```python
from build123d import *

# Parameters (mm, degrees)
BOSS_EXTRUDE1_DEPTH = 20
BOSS_EXTRUDE2_DEPTH = 10
FILLET1_R           = 3
FILLET2_R           = 1
BOSS_EXTRUDE4_DEPTH = 2
CUT_EXTRUDE1_REACH  = 44.805


with BuildPart() as part:
    # Sketch1 → Boss-Extrude1 (new body)
    with BuildSketch(Plane.XY):
        with BuildLine():
            Line((-11.5, 7), (11.5, 7))
            ThreePointArc((11.5, 7), (18.5, 0), (11.5, -7))
            Line((11.5, -7), (-11.5, -7))
            ThreePointArc((-11.5, -7), (-18.5, 0), (-11.5, 7))
        make_face()
        with BuildLine():
            Line((-11.5, 5), (11.5, 5))
            ThreePointArc((11.5, 5), (16.5, 0), (11.5, -5))
            Line((11.5, -5), (-11.5, -5))
            ThreePointArc((-11.5, -5), (-16.5, 0), (-11.5, 5))
        make_face(mode=Mode.SUBTRACT)
    extrude(amount=BOSS_EXTRUDE1_DEPTH)

    # Sketch2 → Boss-Extrude2 (add)
    with BuildSketch(Plane(origin=(0, 0, 0), x_dir=(-1, 0, 0), z_dir=(0, 0, -1))):
        with BuildLine():
            Line((11.25, -7), (6.75, -7))
            ThreePointArc((6.75, -7), (9.829603655, -12.636154321), (8.962619003, -19))
            Line((8.962619003, -19), (11.25, -19))
            Line((11.25, -19), (11.25, -7))
        make_face()
        with BuildLine():
            Line((-11.25, -19), (-8.962619003, -19))
            ThreePointArc((-8.962619003, -19), (-9.829603655, -12.636154321), (-6.75, -7))
            Line((-6.75, -7), (-11.25, -7))
            Line((-11.25, -7), (-11.25, -19))
        make_face()
    extrude(amount=-BOSS_EXTRUDE2_DEPTH)

    # Fillet1
    # the kernel refuses this fillet: 3 mm, written as the material it adds along each edge
    with BuildSketch(Plane(origin=(-11.25, -7, 0), x_dir=(-0.9923889232111901, 0.12314310816174315, 0), z_dir=(0, 0, 1))) as fillet1_piece_1:
        with BuildLine():
            CenterArc((2.655216223, 2.963972865), FILLET1_R, 187.073535236, 74.037985837)
            Line((-0.321950546, 2.594543541), (-0.619667223, 2.557600608))
            Line((-0.619667223, 2.557600608), (-0.297716677, -0.036942932))
            Line((-0.297716677, -0.036942932), (0.036942932, -0.297716677))
            ThreePointArc((0.036942932, -0.297716677), (0.285040163, -0.2669309), (2.145327536, -0.296397287))
            Line((2.145327536, -0.296397287), (2.191681053, 0))
        make_face()
    extrude(amount=10)
    with BuildSketch(Plane(origin=(11.25, -7, 0), x_dir=(0.9923889232111899, 0.12314310816174322, 0), z_dir=(0, 0, 1))) as fillet1_piece_2:
        with BuildLine():
            CenterArc((2.655216223, -2.963972865), FILLET1_R, 98.888478927, 74.037985837)
            Line((-0.321950546, -2.594543541), (-0.619667223, -2.557600608))
            Line((-0.619667223, -2.557600608), (-0.297716677, 0.036942932))
            Line((-0.297716677, 0.036942932), (0.036942932, 0.297716677))
            ThreePointArc((0.036942932, 0.297716677), (0.285040163, 0.2669309), (2.145327536, 0.296397287))
            Line((2.145327536, 0.296397287), (2.191681053, 0))
        make_face()
    extrude(amount=10)

    # Fillet2
    fillet2_edges = [part.edges().sort_by_distance(p)[0] for p in [
        (-6.75, -7, 5),
        (-11.25, -19, 5),
        (6.75, -7, 5),
        (11.25, -19, 5),
    ]]
    fillet(fillet2_edges, radius=FILLET2_R)

    # Sketch3 → Boss-Extrude4 (add)
    with BuildSketch(Plane(origin=(0, 7, 0), x_dir=(1, 0, 0), z_dir=(0, 1, 0))):
        Polygon((-27.5, -20), (27.5, -20), (27.5, 5), (20.5, 5), (20.5, -10), (-20.5, -10), (-20.5, 5), (-27.5, 5), align=None)
    extrude(amount=BOSS_EXTRUDE4_DEPTH)

    # Sketch4 → Cut-Extrude1 (cut, up to next)
    with BuildSketch(Plane.XZ.offset(-7), mode=Mode.PRIVATE) as cut_extrude1_sk1:
        with BuildLine():
            Line((-24, 17.5), (-24, -2.5))
            ThreePointArc((-24, -2.5), (-24.5, -3), (-25, -2.5))
            Line((-25, -2.5), (-25, 17.5))
            ThreePointArc((-25, 17.5), (-24.5, 18), (-24, 17.5))
        make_face()
    cut_extrude1_tool1 = extrude(cut_extrude1_sk1.sketch, amount=-CUT_EXTRUDE1_REACH, mode=Mode.PRIVATE) & part.part
    cut_extrude1 = cut_extrude1_tool1.solids().sort_by_distance((-24.5, 7, 7.5))[0]
    add(cut_extrude1, mode=Mode.SUBTRACT)

    # Mirror1: Cut-Extrude1 across plane
    add(cut_extrude1.mirror(Plane(origin=(0, 0, 0), x_dir=(0, 0, 1), z_dir=(1, 0, 0))), mode=Mode.SUBTRACT)


solid = part.part
```
Work out the finished part from the listing and answer in its coordinate system (mm). A direction names the side the tool comes from. Give positions to 0.01 mm unless a question says otherwise; leave off trailing zeros. Loops run counter-clockwise (first coordinate to the right, second up) from the corner with the lowest first, then second, coordinate; pieces in that order, holes last. Notation, with made-up numbers: (-7.5, 10) - (26.5, 10) arc R24 cw to (26.5, 34) - close; hole circle Ø9 at (-39, -19). An arc over 180 degrees is marked (long way). One line per question, with ' | ' between items.
(1) The part is cut by section A-A (y = -14.5). Write down the section's boundary in (x, z).
Recorded:
outline: (-11.25, 0) - (-10, 0) - (-10, 10) - (-11.25, 10) - close; (10, 0) - (11.25, 0) - (11.25, 10) - (10, 10) - close
(2) The part is cut by section B-B (z = 12.5). Write down the section's boundary in (x, y).
Recorded:
outline: (-27.5, 7) - (-25, 7) - (-25, 9) - (-27.5, 9) - close; (-24, 7) - (-11.5, 7) arc R7 ccw to (-11.5, -7) - (11.5, -7) arc R7 ccw to (11.5, 7) - (24, 7) - (24, 9) - (-24, 9) - close; (25, 7) - (27.5, 7) - (27.5, 9) - (25, 9) - close; hole (-11.5, -5) - (11.5, -5) arc R5 ccw to (11.5, 5) - (-11.5, 5) arc R5 ccw to start
(3) The part is cut by section C-C (y = 0). Write down the section's boundary in (x, z).
Recorded:
outline: (-18.5, 0) - (-16.5, 0) - (-16.5, 20) - (-18.5, 20) - close; (16.5, 0) - (18.5, 0) - (18.5, 20) - (16.5, 20) - close
(4) A tool of negligible diameter and unlimited length cuts with its end or side. For faces 5 (the face through (-24.5, 8, 18)), 6 (the face through (16.5, 0.1, 9.9)), 7 (the face through (-27.5, 8, 7)), from which of +Z, -Z, +X, -X, +Y, -Y can it reach the whole face along a straight path? Write none if from no direction.
Recorded:
face 5: +Y, -Y | face 6: +Z, -Z | face 7: +Z, -Z, -X, +Y, -Y
(5) The part is cut by section D-D (z = 8.5). Count the separate pieces of the cut face and the enclosed holes in it, then the cut area to 3 significant figures.
Recorded:
separate pieces: 5 | enclosed holes: 1 | area: 242 mm²
(6) Straight lines are drawn through the part: probe 1 along Y at (x, z) = (-11, 15); probe 2 along Y at (x, z) = (3, 4); probe 3 along Y at (x, z) = (-15.5, 17.5). For each, find the intervals that lie inside material, in ascending order.
Recorded:
probe 1: y = -7 to -5, 5 to 9 | probe 2: y = -7 to -5, 5 to 7 | probe 3: y = -5.74 to -3, 3 to 5.74, 7 to 9
(7) The mould has two halves that part along Z. Classify faces 1 (the face through (24, 8, -5)), 2 (the face through (-11.25, -14, 5)), 3 (the face through (-24.5, 8, -3)), 4 (the face through (0, 6, 20)): +Z half, -Z half, draft (parallel to the pull), parting line (faces both ways), or undercut.
Recorded:
face 1: -Z half | face 2: draft | face 3: undercut | face 4: +Z half
(8) Each of these flat-tipped pins is pushed along its axis until it touches: pin 1 Ø1.5 at (x, z) = (21, -0.5) entering from -Y; pin 2 Ø12 at (y, z) = (-10, 14.5) entering from -X; pin 3 Ø1 at (x, y) = (1.5, 8) entering from -Z. Where does it stop, or does it pass through?
Recorded:
pin 1: stops at y = 7 | pin 2: stops at x = -17.24 | pin 3: stops at z = 10
